The listing builds one solid part. Answer for the finished solid, in the listing's coordinates (mm). Give positions to 0.01 mm unless a question says otherwise; leave off trailing zeros. Order: outer loops, then holes, each group sorted by start corner. A loop starts at its lowest first (then second) coordinate and runs counter-clockwise, first axis right, second up. Notation, with made-up numbers: (37, 24.25) -> (46, 24.25) arc R11 cw to (46, 36.25) -> close; hole circle Ø5 at (23.5, 57). An arc over 180 degrees is marked (long way). Write item = value, one per line. Start each with the question number.
```python
from build123d import *

# Parameters (mm, degrees)
EXTRUDE_1_DEPTH   = 2
HOLE_WIZARD_M81_D = 9
CHAMFER_1_SIZE    = 2


with BuildPart() as part:
    # Эскиз1 → Бобышка-Вытянуть1 (new body)
    with BuildSketch(Plane(origin=(0, 0, 0), x_dir=(1, 0, 0), z_dir=(0, 0, -1))):
        Polygon((0, 0), (0, 200), (150, 200), (150, 100), (100, 100), (100, 0), align=None)
    extrude(amount=EXTRUDE_1_DEPTH)

    # Отверстие с зазором M81 (through all)
    with Locations(Plane(origin=(0, 0, -2), x_dir=(1, 0, 0), z_dir=(0, 0, -1))):
        with Locations((25, 175), (25, 125), (25, 75), (25, 25), (75, 175), (75, 125), (75, 75), (75, 25), (125, 175), (125, 125)):
            Hole(HOLE_WIZARD_M81_D / 2)

    # Фаска1
    chamfer_1_edges = [part.edges().sort_by_distance(p)[0] for p in [
        (0, 0, -1),
        (0, -200, -1),
        (150, -200, -1),
        (150, -100, -1),
        (100, 0, -1),
    ]]
    chamfer(chamfer_1_edges, length=CHAMFER_1_SIZE)


solid = part.part
```
Item 1: The mould has two halves that part along X. Classify faces 1 (the flat face through (59, -101, 0)), 2 (the cylindrical face through (72.581, -28.794, -0.986)): +X half, -X half, draft (parallel to the pull), parting line (faces both ways), or undercut.
Item 2: A cutting plane is placed at C-C, the plane x = 75. Write down the section's boundary in (y, z).
Item 3: A cutting plane is placed at D-D, the plane y = -25. Write down the section's boundary in (x, z), plus the area to 3 significant figures.
Item 4: Flat-ended cylindrical pins translate along their axes: pin 1 (8 mm diameter, centred on x = 25, y = -75, fed in from -Z); pin 2 (0.6 mm diameter, centred on x = 134.5, z = -1.5, fed in from +Y); pin 3 (0.6 mm diameter, centred on y = -75, z = -1, fed in from +X). Find the tip coordinate at first contact, or state that the pin passes through.
Item 5: Consider L1, parallel to X at y = -175, z = -0.35; L2, parallel to Y at x = 125, z = -1.2; L3, parallel to Y at x = 25, z = -0.75. Determine where each line is inside the solid, lowest interval first. Write a range as from..to.
Item 6: A cutting plane is placed at B-B, the plane z = -1. Count the separate pieces of the cut face and the enclosed holes in it, plus the area to 3 significant figures.
Item 7: A cutting plane is placed at A-A, the plane y = -175. Write down the section's boundary in (x, z).
Check values:
q1.face_1 = draft
q1.face_2 = undercut
q2.outline = (-200, -2) -> (-179.5, -2) -> (-179.5, 0) -> (-200, 0) -> close; (-170.5, -2) -> (-129.5, -2) -> (-129.5, 0) -> (-170.5, 0) -> close; (-120.5, -2) -> (-79.5, -2) -> (-79.5, 0) -> (-120.5, 0) -> close; (-70.5, -2) -> (-29.5, -2) -> (-29.5, 0) -> (-70.5, 0) -> close; (-20.5, -2) -> (0, -2) -> (0, 0) -> (-20.5, 0) -> close
q3.outline = (0, -2) -> (20.5, -2) -> (20.5, 0) -> (0, 0) -> close; (29.5, -2) -> (70.5, -2) -> (70.5, 0) -> (29.5, 0) -> close; (79.5, -2) -> (100, -2) -> (100, 0) -> (79.5, 0) -> close
q3.area = 164 mm^2
q4.pin_1 = through
q4.pin_2 = -100
q4.pin_3 = 100
q5.L1 = 0..20.5, 29.5..70.5, 79.5..120.5, 129.5..150
q5.L2 = -200..-179.5, -170.5..-129.5, -120.5..-100
q5.L3 = -200..-179.5, -170.5..-129.5, -120.5..-79.5, -70.5..-29.5, -20.5..0
q6.separate_pieces = 1
q6.enclosed_holes = 10
q6.area = 24,400 mm^2
q7.outline = (0, -2) -> (20.5, -2) -> (20.5, 0) -> (0, 0) -> close; (29.5, -2) -> (70.5, -2) -> (70.5, 0) -> (29.5, 0) -> close; (79.5, -2) -> (120.5, -2) -> (120.5, 0) -> (79.5, 0) -> close; (129.5, -2) -> (150, -2) -> (150, 0) -> (129.5, 0) -> close
